Model file for the job. Use its own axes, mm. A direction names the side the tool comes from. Round coordinates to 2 decimals unless told otherwise and drop trailing zeros. Loops run counter-clockwise (first coordinate to the right, second up) from the corner with the lowest first, then second, coordinate; pieces in that order, holes last. Notation, with made-up numbers: M 61.25,42.5 L 84.25,42.5 A23 cw 84.25,59.5 Z; hole C -5.75,26 d3. An arc over 180 degrees is marked long. Answer in a Markdown table with one row per item.
from build123d import *

# Parameters (mm, degrees)
SKETCH1_W           = 200
SKETCH1_H           = 160
BOSS_EXTRUDE3_DEPTH = 10
SKETCH3_R           = 3.75
SKETCH3_W           = 160
SKETCH3_H           = 120
CUT_EXTRUDE2_DEPTH  = 6
SKETCH6_R           = 3.75
CUT_EXTRUDE4_DEPTH  = 129.202964084
SKETCH7_W           = 30
SKETCH7_H           = 160
BOSS_EXTRUDE4_DEPTH = 2


with BuildPart() as part:
    # Sketch1 → Boss-Extrude3 (new body)
    with BuildSketch(Plane(origin=(0, 0, 0), x_dir=(1, 0, 0), z_dir=(0, 1, 0))):
        Rectangle(SKETCH1_W, SKETCH1_H)
    extrude(amount=BOSS_EXTRUDE3_DEPTH)

    # Sketch3 → Cut-Extrude2 (cut)
    with BuildSketch(Plane(origin=(0, 10, 0), x_dir=(1, 0, 0), z_dir=(0, 1, 0))):
        with Locations(Location((-90, 70, 0), (0, 0, 270))):
            Circle(SKETCH3_R)
        with Locations(Location((90, -70, 0), (0, 0, 270))):
            Circle(SKETCH3_R)
        with Locations(Location((90, 70, 0), (0, 0, 270))):
            Circle(SKETCH3_R)
        with Locations(Location((-90, -70, 0), (0, 0, 270))):
            Circle(SKETCH3_R)
        Rectangle(SKETCH3_W, SKETCH3_H)
    extrude(amount=-CUT_EXTRUDE2_DEPTH, mode=Mode.SUBTRACT)

    # Sketch6 → Cut-Extrude4 (cut, through all)
    with BuildSketch(Plane(origin=(0, 4, 0), x_dir=(1, 0, 0), z_dir=(0, 1, 0))):
        with Locations(Location((-90, 70, 0), (0, 0, 270))):
            Circle(SKETCH6_R)
        with Locations(Location((90, 70, 0), (0, 0, 270))):
            Circle(SKETCH6_R)
        with Locations(Location((90, -70, 0), (0, 0, 270))):
            Circle(SKETCH6_R)
        with Locations(Location((-90, -70, 0), (0, 0, 270))):
            Circle(SKETCH6_R)
    extrude(amount=-CUT_EXTRUDE4_DEPTH, mode=Mode.SUBTRACT)

    # Sketch7 → Boss-Extrude4 (add)
    with BuildSketch(Plane(origin=(0, 0, 0), x_dir=(-1, 0, 0), z_dir=(0, -1, 0))):
        Rectangle(SKETCH7_W, SKETCH7_H)
        with Locations((60, 0)):
            Rectangle(SKETCH7_W, SKETCH7_H)
        with Locations((-60, 0)):
            Rectangle(SKETCH7_W, SKETCH7_H)
    extrude(amount=BOSS_EXTRUDE4_DEPTH)


solid = part.part
1. Wall check: probe 1 along X at (y, z) = (4.75, -70); probe 2 along X at (y, z) = (8, -54.5); probe 3 along Z at (x, y) = (-88.5, 8). Give the ranges that are in metal, low to high.
Verdict:
| item | result |
|---|---|
| probe 1 | x = -100 to -93.75, -86.25 to 86.25, 93.75 to 100 |
| probe 2 | x = -100 to -80, 80 to 100 |
| probe 3 | z = -80 to -73.44, -66.56 to 66.56, 73.44 to 80 |
2. Tool access for faces 4 (the flat face through (-88, 0, -1)), 5 (the flat face through (-1, 4, -80)), 6 (the flat face through (-30, 0, -1)), 7 (the flat face through (80, 7, 1)), 8 (the flat face through (87, 0, -1)): list every direction of +Z, -Z, +X, -X, +Y, -Y with a clear straight run to the whole face (end or side of a thin tool).
Verdict:
| item | result |
|---|---|
| face 4 | +Z, -Z, -X, -Y |
| face 5 | -Z, +X, -X, +Y, -Y |
| face 6 | +Z, -Z, -Y |
| face 7 | +Y |
| face 8 | +Z, -Z, +X, -Y |
3. Pin check, flat tips, straight feed: pin 1 (12 mm diameter, centred on x = -51.5, z = -7, fed in from +Y); pin 2 (7.5 mm diameter, centred on x = 93.5, z = 11.5, fed in from -Y); pin 3 (0.6 mm diameter, centred on y = -0.5, z = -36, fed in from -X). Stop position of each tip, or through.
Verdict:
| item | result |
|---|---|
| pin 1 | stops at y = 4 |
| pin 2 | stops at y = 0 |
| pin 3 | stops at x = -75 |
4. Saw through at D-D (z = -12). Write the cut outline in (x, y), and give its area (3 significant figures).
Verdict:
| item | result |
|---|---|
| outline | M -100,0 L -75,0 L -75,-2 L -45,-2 L -45,0 L -15,0 L -15,-2 L 15,-2 L 15,0 L 45,0 L 45,-2 L 75,-2 L 75,0 L 100,0 L 100,10 L 80,10 L 80,4 L -80,4 L -80,10 L -100,10 Z |
| area | 1,220 mm² |
5. Saw through at A-A (x = -90). Write the cut outline in (y, z).
Verdict:
| item | result |
|---|---|
| outline | M 0,-80 L 10,-80 L 10,-73.75 L 0,-73.75 Z; M 0,-66.25 L 10,-66.25 L 10,66.25 L 0,66.25 Z; M 0,73.75 L 10,73.75 L 10,80 L 0,80 Z |
6. Mould opens along X. For faces 1 (the flat face through (-1, 4, -1)), 2 (the flat face through (-100, 5, 1)), 3 (the flat face through (60, -2, -1)) say: +X half, -X half, draft (parallel to the pull), parting line (faces both ways), or undercut.
Verdict:
| item | result |
|---|---|
| face 1 | undercut |
| face 2 | -X half |
| face 3 | draft |
7. Saw through at B-B (z = 70). Write the cut outline in (x, y).
Verdict:
| item | result |
|---|---|
| outline | M -100,0 L -93.75,0 L -93.75,10 L -100,10 Z; M -86.25,0 L -75,0 L -75,-2 L -45,-2 L -45,0 L -15,0 L -15,-2 L 15,-2 L 15,0 L 45,0 L 45,-2 L 75,-2 L 75,0 L 86.25,0 L 86.25,10 L -86.25,10 Z; M 93.75,0 L 100,0 L 100,10 L 93.75,10 Z |
8. Saw through at C-C (x = -65.5). Write the cut outline in (y, z), and give its area (3 significant figures).
Verdict:
| item | result |
|---|---|
| outline | M -2,-80 L 10,-80 L 10,-60 L 4,-60 L 4,60 L 10,60 L 10,80 L -2,80 Z |
| area | 1,200 mm² |
